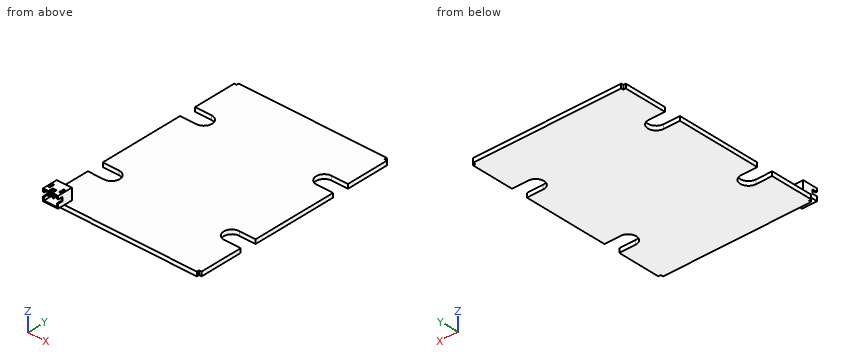
from build123d import *

# Parameters (mm, degrees)
PAD_DEPTH       = 1.7
SKETCH008_W     = 6.1
SKETCH008_H     = 6.1
PAD003_DEPTH    = 4.6
SKETCH014_W     = 5.16
SKETCH014_H     = 3.66
SKETCH014_W_2   = 0.48
SKETCH014_H_2   = 0.48
POCKET003_DEPTH = 5.44
SKETCH015_W     = 0.47
SKETCH015_H     = 1.56
SKETCH015_W_2   = 1.56
SKETCH015_H_2   = 0.47
POCKET004_DEPTH = 2
SKETCH016_W     = 0.6
SKETCH016_H     = 2.02
POCKET005_DEPTH = 1


with BuildPart() as part:
    # Sketch → Pad (new body)
    with BuildSketch(Plane.XY):
        with BuildLine():
            Line((0, 0), (30, 0))
            Line((30, 0), (30, 1))
            Line((30, 1), (31, 1))
            Line((31, 1), (31, 18.27))
            Line((31, 18.27), (24.4, 18.27))
            ThreePointArc((24.4, 24.87), (21.1, 21.57), (24.4, 18.27))
            Line((24.4, 24.87), (31, 24.87))
            Line((31, 24.87), (31, 59.13))
            Line((31, 59.13), (24.4, 59.13))
            ThreePointArc((24.4, 65.73), (21.1, 62.43), (24.4, 59.13))
            Line((24.4, 65.73), (31, 65.73))
            Line((31, 65.73), (31, 83))
            Line((30, 83), (31, 83))
            Line((30, 84), (30, 83))
            Line((30, 84), (0, 84))
            Line((0, 84), (-30, 84))
            Line((-30, 84), (-30, 83))
            Line((-30, 83), (-31, 83))
            Line((-31, 83), (-31, 65.73))
            Line((-31, 65.73), (-24.4, 65.73))
            ThreePointArc((-24.4, 59.13), (-21.1, 62.43), (-24.4, 65.73))
            Line((-24.4, 59.13), (-31, 59.13))
            Line((-31, 59.13), (-31, 24.87))
            Line((-31, 24.87), (-24.4, 24.87))
            ThreePointArc((-24.4, 18.27), (-21.1, 21.57), (-24.4, 24.87))
            Line((-24.4, 18.27), (-31, 18.27))
            Line((-31, 18.27), (-31, 1))
            Line((-31, 1), (-30, 1))
            Line((-30, 1), (-30, 0))
            Line((-30, 0), (0, 0))
        make_face()
    extrude(amount=PAD_DEPTH)

    # Sketch008 → Pad003 (new body)
    with BuildSketch(Plane.XY.offset(1.7)):
        with Locations((-26.82, 0.25)):
            Rectangle(SKETCH008_W, SKETCH008_H)
    extrude(amount=PAD003_DEPTH)

    # Sketch014 → Pocket003 (cut)
    with BuildSketch(Plane.XZ.offset(2.8)):
        with Locations((-26.82, 4)):
            Rectangle(SKETCH014_W, SKETCH014_H)
        with Locations((-27.96, 4.76)):
            Rectangle(SKETCH014_W_2, SKETCH014_H_2, mode=Mode.SUBTRACT)
        with Locations((-25.86, 4.76)):
            Rectangle(SKETCH014_W_2, SKETCH014_H_2, mode=Mode.SUBTRACT)
    extrude(amount=-POCKET003_DEPTH, mode=Mode.SUBTRACT)

    # Sketch015 → Pocket004 (cut)
    with BuildSketch(Plane.XZ.offset(2.8)):
        with Locations((-29.635, 4.22)):
            Rectangle(SKETCH015_W, SKETCH015_H)
        with Locations((-24.005, 4.22)):
            Rectangle(SKETCH015_W, SKETCH015_H)
        with Locations((-26.91, 6.065)):
            Rectangle(SKETCH015_W_2, SKETCH015_H_2)
    extrude(amount=-POCKET004_DEPTH, mode=Mode.SUBTRACT)

    # Sketch016 → Pocket005 (cut)
    with BuildSketch(Plane.XY.offset(6.3)):
        with Locations((-29.01, -0.01)):
            Rectangle(SKETCH016_W, SKETCH016_H)
        with Locations((-24.63, -0.01)):
            Rectangle(SKETCH016_W, SKETCH016_H)
    extrude(amount=-POCKET005_DEPTH, mode=Mode.SUBTRACT)


solid = part.part
The listing builds one solid part. Answer for the finished solid, in the listing's coordinates (mm). Give positions to 0.01 mm unless a question says otherwise; leave off trailing zeros. Order: outer loops, then holes, each group sorted by start corner. A loop starts at its lowest first (then second) coordinate and runs counter-clockwise, first axis right, second up. Notation, with made-up numbers: (50, 25) -> (91, 25) arc R23 cw to (91, 57) -> close; hole circle Ø11 at (64.5, 32.25). An arc over 180 degrees is marked (long way). Put each result on its own line as item: value.
Item 1: A cutting plane is placed at C-C on x = -9. Give the vertices of the cut face in (y, z).
Established:
outline: (0, 0) -> (84, 0) -> (84, 1.7) -> (0, 1.7) -> close
Item 2: A cutting plane is placed at B-B on y = 16.5. Give the vertices of the cut face in (x, z).
Established:
outline: (-31, 0) -> (31, 0) -> (31, 1.7) -> (-31, 1.7) -> close
Item 3: Given P1, Ø0.5, axis at y = -0.5, z = 4.5, coming from the -X side; P2, Ø10, axis at x = -3, y = 27, coming from the +Z side; P3, Ø3.5, axis at x = -27, z = 4.5, coming from the +Y side; P4, Ø1, axis at x = 3.5, z = 4, coming from the +Y side, each flat-ended and moving along its own axis, determine where each tip first touches the part or whether it passes through.
Established:
P1: stops at x = -29.87
P2: stops at z = 1.7
P3: stops at y = 3.3
P4: passes through
Item 4: Straight lines are drawn through the part: line 1 (Z direction, x = -26, y = 1.5); line 2 (Y direction, x = -27.5, z = 1); line 3 (Z direction, x = 16.5, y = 64.5). For each, find the intervals that lie inside material, in ascending order.
Established:
line 1: z = 0 to 2.17, 4.52 to 5, 5.83 to 6.3
line 2: y = 0 to 18.27, 24.87 to 59.13, 65.73 to 84
line 3: z = 0 to 1.7
Item 5: A cutting plane is placed at A-A on x = -22.5. Give the vertices of the cut face in (y, z).
Established:
outline: (0, 0) -> (18.87, 0) -> (18.87, 1.7) -> (0, 1.7) -> close; (24.27, 0) -> (59.73, 0) -> (59.73, 1.7) -> (24.27, 1.7) -> close; (65.13, 0) -> (84, 0) -> (84, 1.7) -> (65.13, 1.7) -> close
